CAD build for the part. Positions are in the model's coordinates, mm. Coordinates: 2 decimals unless noted, no trailing zeros. Loops run counter-clockwise (first coordinate to the right, second up) from the corner with the lowest first, then second, coordinate; pieces in that order, holes last. Notation, with made-up numbers: (13, 81) -> (24, 81) arc R33 ccw to (24, 120) -> close; hole circle Ø11 at (25, 54). An arc over 180 degrees is marked (long way). Answer as a JSON object with one key per item and string values. Group by question number.
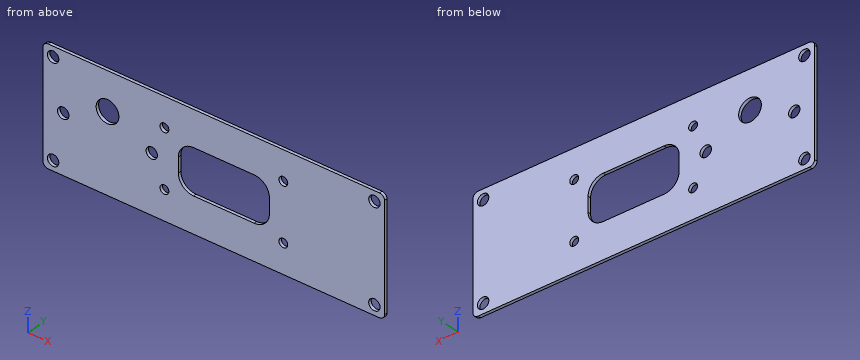
from build123d import *

# Parameters (mm, degrees)
BASE_R      = 2.25
BASE_R_2    = 1.75
BASE_R_3    = 4.5
SHEET_DEPTH = 1.2192


with BuildPart() as part:
    # BASE → SHEET (new body)
    with BuildSketch(Plane(origin=(0, 0, 0), x_dir=(1, 0, 0), z_dir=(0, 1, 0))):
        with BuildLine():
            Line((65.5, -23.25), (-65.5, -23.25))
            ThreePointArc((-65.5, -23.25), (-66.914213562, -22.664213562), (-67.5, -21.25))
            Line((-67.5, -21.25), (-67.5, 21.25))
            ThreePointArc((-67.5, 21.25), (-66.914213562, 22.664213562), (-65.5, 23.25))
            Line((-65.5, 23.25), (65.5, 23.25))
            ThreePointArc((65.5, 23.25), (66.914213562, 22.664213562), (67.5, 21.25))
            Line((67.5, 21.25), (67.5, -21.25))
            ThreePointArc((67.5, -21.25), (66.914213562, -22.664213562), (65.5, -23.25))
        make_face()
        with Locations(Location((-59.5, 0, 0), (0, 0, 270))):
            Circle(BASE_R, mode=Mode.SUBTRACT)
        with Locations(Location((-24.5, 0, 0), (0, 0, 270))):
            Circle(BASE_R, mode=Mode.SUBTRACT)
        with Locations(Location((-63.5, 19.25, 0), (0, 0, 270))):
            Circle(BASE_R, mode=Mode.SUBTRACT)
        with Locations(Location((-63.5, -19.25, 0), (0, 0, 270))):
            Circle(BASE_R, mode=Mode.SUBTRACT)
        with Locations(Location((63.5, -19.25, 0), (0, 0, 270))):
            Circle(BASE_R, mode=Mode.SUBTRACT)
        with Locations(Location((63.5, 19.25, 0), (0, 0, 270))):
            Circle(BASE_R, mode=Mode.SUBTRACT)
        with Locations(Location((-19.5, 11.5, 0), (0, 0, 270))):
            Circle(BASE_R_2, mode=Mode.SUBTRACT)
        with Locations(Location((27.5, 11.5, 0), (0, 0, 270))):
            Circle(BASE_R_2, mode=Mode.SUBTRACT)
        with Locations(Location((27.5, -11.5, 0), (0, 0, 270))):
            Circle(BASE_R_2, mode=Mode.SUBTRACT)
        with Locations(Location((-19.5, -11.5, 0), (0, 0, 270))):
            Circle(BASE_R_2, mode=Mode.SUBTRACT)
        with Locations(Location((-42, -8, 0), (0, 0, 270))):
            Circle(BASE_R_3, mode=Mode.SUBTRACT)
        with BuildLine():
            Line((-8, -9), (16, -9))
            ThreePointArc((16, -9), (20.242640687, -7.242640687), (22, -3))
            Line((22, -3), (22, 3))
            ThreePointArc((22, 3), (20.242640687, 7.242640687), (16, 9))
            Line((16, 9), (-8, 9))
            ThreePointArc((-8, 9), (-12.242640687, 7.242640687), (-14, 3))
            Line((-14, 3), (-14, -3))
            ThreePointArc((-14, -3), (-12.242640687, -7.242640687), (-8, -9))
        make_face(mode=Mode.SUBTRACT)
    extrude(amount=SHEET_DEPTH)


solid = part.part
Item 1: Band-saw the part on C-C, the plane y = 0.8. Count the separate pieces of the cut face and the enclosed holes in it, and give its area (3 significant figures).
Item 2: Band-saw the part on D-D, the plane z = 0. List the corners of the cut face in (x, y).
Item 3: Band-saw the part on A-A, the plane x = -24.5. List the corners of the cut face in (y, z), and give its area (3 significant figures).
Item 4: Flat gauge pin, fed straight in: P1, Ø2.5, axis at x = -63.5, z = -19.25, coming from the -Y side. Where does the tip first touch, or does it go through?
Item 5: Band-saw the part on B-B, the plane z = -19.25. List the corners of the cut face in (x, y), and give its area (3 significant figures).
Item 6: Drill centre lines: L1, parallel to X at y = 0.7, z = 19; L2, parallel to X at y = 0.5, z = 0; L3, parallel to X at y = 0.5, z = -11.5. Where is each one in solid material? Low to high.
Reply:
{
 "1": {"separate pieces": "1", "enclosed holes": "12", "area": "5,460 mm²"},
 "2": {"outline": "(-67.5, 0) -> (-61.75, 0) -> (-61.75, 1.22) -> (-67.5, 1.22) -> close; (-57.25, 0) -> (-26.75, 0) -> (-26.75, 1.22) -> (-57.25, 1.22) -> close; (-22.25, 0) -> (-14, 0) -> (-14, 1.22) -> (-22.25, 1.22) -> close; (22, 0) -> (67.5, 0) -> (67.5, 1.22) -> (22, 1.22) -> close"},
 "3": {"outline": "(0, -23.25) -> (1.22, -23.25) -> (1.22, -2.25) -> (0, -2.25) -> close; (0, 2.25) -> (1.22, 2.25) -> (1.22, 23.25) -> (0, 23.25) -> close", "area": "51.2 mm²"},
 "4": {"P1": "through"},
 "5": {"outline": "(-67.5, 0) -> (-65.75, 0) -> (-65.75, 1.22) -> (-67.5, 1.22) -> close; (-61.25, 0) -> (61.25, 0) -> (61.25, 1.22) -> (-61.25, 1.22) -> close; (65.75, 0) -> (67.5, 0) -> (67.5, 1.22) -> (65.75, 1.22) -> close", "area": "154 mm²"},
 "6": {"L1": "-67.5 to -65.74, -61.26 to 61.26, 65.74 to 67.5", "L2": "-67.5 to -61.75, -57.25 to -26.75, -22.25 to -14, 22 to 67.5", "L3": "-67.5 to -21.25, -17.75 to 25.75, 29.25 to 67.5"}
}
